```python
from build123d import *

# Parameters (mm, degrees)
SKETCH1_W             = 20
SKETCH1_H             = 12
BOSS_EXTRUDE1_DEPTH   = 22
M6X1_0_TAPPED_HOLE1_D = 5
SKETCH7_W             = 2
SKETCH7_H             = 2
CUT_EXTRUDE2_DEPTH    = 46.519226707
FILLET1_RADIUS        = 10
FILLET1_LENGTH        = 12
FILLET2_RADIUS        = 10
FILLET2_LENGTH        = 12


with BuildPart() as part:
    # Sketch1 → Boss-Extrude1 (new, symmetric)
    with BuildSketch(Plane.XY):
        Rectangle(SKETCH1_W, SKETCH1_H)
    extrude(amount=BOSS_EXTRUDE1_DEPTH, both=True)

    # M6x1.0 Tapped Hole1 (through all)
    with Locations(Plane(origin=(0, 6, 0), x_dir=(1, 0, 0), z_dir=(0, 1, 0))):
        with Locations((0, -15), (0, 0), (0, 15)):
            Hole(M6X1_0_TAPPED_HOLE1_D / 2)

    # Sketch7 → Cut-Extrude2 (cut, through all)
    with BuildSketch(Plane(origin=(0, 0, -22), x_dir=(-1, 0, 0), z_dir=(0, 0, -1))):
        with Locations((0, 5)):
            Rectangle(SKETCH7_W, SKETCH7_H)
    extrude(amount=-CUT_EXTRUDE2_DEPTH, mode=Mode.SUBTRACT)

    # Fillet1: full round fillet: the end face becomes a half cylinder, R = half its width
    fillet1_face = Plane((0, 0, -22), x_dir=(0, -1, 0), z_dir=(0, 0, -1))  # on the end face: x along it, z out of the body
    fillet1_slab = fillet1_face.offset(-FILLET1_RADIUS / 2) * Box(FILLET1_LENGTH, 2 * FILLET1_RADIUS, FILLET1_RADIUS, mode=Mode.PRIVATE)  # the body's end, R deep
    fillet1_round = Plane((0, 0, -12), x_dir=(0, 0, -1), z_dir=(0, -1, 0)) * Cylinder(FILLET1_RADIUS, FILLET1_LENGTH, mode=Mode.PRIVATE)  # its axis R under the face
    add(fillet1_slab - fillet1_round, mode=Mode.SUBTRACT)

    # Fillet2: full round fillet: the end face becomes a half cylinder, R = half its width
    fillet2_face = Plane((0, 0, 22), x_dir=(0, 1, 0), z_dir=(0, 0, 1))  # on the end face: x along it, z out of the body
    fillet2_slab = fillet2_face.offset(-FILLET2_RADIUS / 2) * Box(FILLET2_LENGTH, 2 * FILLET2_RADIUS, FILLET2_RADIUS, mode=Mode.PRIVATE)  # the body's end, R deep
    fillet2_round = Plane((0, 0, 12), x_dir=(0, 0, 1), z_dir=(0, 1, 0)) * Cylinder(FILLET2_RADIUS, FILLET2_LENGTH, mode=Mode.PRIVATE)  # its axis R under the face
    add(fillet2_slab - fillet2_round, mode=Mode.SUBTRACT)


solid = part.part
```
Geometry: final body of the model. Coordinates: model frame, mm. A direction names the side the tool comes from. Give positions to 0.01 mm unless a question says otherwise; leave off trailing zeros. Loops run counter-clockwise (first coordinate to the right, second up) from the corner with the lowest first, then second, coordinate; pieces in that order, holes last. Notation, with made-up numbers: (77.25, 48) -> (111.25, 48) arc R14 cw to (111.25, 56) -> close; hole circle Ø9 at (81, 9.25). An arc over 180 degrees is marked (long way). Return JSON: item names as keys, results as strings.
Item 1: Pin query (flat end, axial travel): P1, Ø2, axis at x = -6, y = 3, coming from the +Z side; P2, Ø0.6, axis at y = 5.5, z = 19, coming from the +X side; P3, Ø3, axis at x = 0, z = -15, coming from the +Y side; P4, Ø1.6, axis at x = 0, z = -7.5, coming from the +Y side. Return the tip coordinate at first contact, or that it passes through.
Filled in:
{"P1": "z = 20.66", "P2": "x = 7.42", "P3": "through", "P4": "y = 4"}
Item 2: Line query: line 1 (Z direction, x = 0, y = 1.5); line 2 (X direction, y = 4.5, z = 4.5); line 3 (X direction, y = -0.75, z = 16.5). Output: solid intervals per line, ascending.
Filled in:
{"line 1": "-22 to -17.5, -12.5 to -2.5, 2.5 to 12.5, 17.5 to 22", "line 2": "-10 to -1, 1 to 10", "line 3": "-8.93 to -2, 2 to 8.93"}
Item 3: Section A-A, the plane z = 0. Output: boundary loops of the cut face in (x, y).
Filled in:
{"outline": "(-10, -6) -> (-2.5, -6) -> (-2.5, 6) -> (-10, 6) -> close; (2.5, -6) -> (10, -6) -> (10, 6) -> (2.5, 6) -> close"}
Item 4: Section C-C, the plane y = 5. Output: boundary loops of the cut face in (x, z).
Filled in:
{"outline": "(-10, -12) arc R10 ccw to (-1, -21.95) -> (-1, -17.29) arc R2.5 cw to (-1, -12.71) -> (-1, -2.29) arc R2.5 cw to (-1, 2.29) -> (-1, 12.71) arc R2.5 cw to (-1, 17.29) -> (-1, 21.95) arc R10 ccw to (-10, 12) -> close; (1, -21.95) arc R10 ccw to (10, -12) -> (10, 12) arc R10 ccw to (1, 21.95) -> (1, 17.29) arc R2.5 cw to (1, 12.71) -> (1, 2.29) arc R2.5 cw to (1, -2.29) -> (1, -12.71) arc R2.5 cw to (1, -17.29) -> close"}
Item 5: Mould query, pull axis Z, two halves, no side actions, for faces 3 (the flat face through (1, 5, 20)), 4 (the cylindrical face through (-2.31, -0.08, -14.04)), 5 (the cylindrical face through (0, 0, 22)), 6 (the cylindrical face through (-2.385, -0.084, -0.751)). Classes: released by +Z, released by -Z, zero draft, split by the parting line, or undercut.
Filled in:
{"face 3": "zero draft", "face 4": "undercut", "face 5": "released by +Z", "face 6": "undercut"}
Item 6: Section B-B, the plane x = 0. Output: boundary loops of the cut face in (y, z).
Filled in:
{"outline": "(-6, -22) -> (4, -22) -> (4, -17.5) -> (-6, -17.5) -> close; (-6, -12.5) -> (4, -12.5) -> (4, -2.5) -> (-6, -2.5) -> close; (-6, 2.5) -> (4, 2.5) -> (4, 12.5) -> (-6, 12.5) -> close; (-6, 17.5) -> (4, 17.5) -> (4, 22) -> (-6, 22) -> close"}
Item 7: Section D-D, the plane y = -0.75. Output: boundary loops of the cut face in (x, z), plus the area to 3 significant figures.
Filled in:
{"outline": "(-10, -12) arc R10 ccw to (10, -12) -> (10, 12) arc R10 ccw to (-10, 12) -> close; hole circle Ø5 at (0, -15); hole circle Ø5 at (0, 0); hole circle Ø5 at (0, 15)", "area": "735 mm^2"}
Item 8: Access query for faces 1 (the cylindrical face through (0, 0, -22)), 2 (the flat face through (-1, 5, 20)). Directions: +Z, -Z, +X, -X, +Y, -Y. A direction counts if a zero-diameter tool reaches every point of the face in a straight line with its end or side. Return the directions, or none.
Filled in:
{"face 1": "-Z, +Y, -Y", "face 2": "+Z, -Z, +Y"}
